Design review of the part built by this model. Coordinates are the model's own, in mm. A direction names the side the tool comes from. Coordinates: 2 decimals unless noted, no trailing zeros. Loops run counter-clockwise (first coordinate to the right, second up) from the corner with the lowest first, then second, coordinate; pieces in that order, holes last. Notation, with made-up numbers: (14, -33) -> (42, -33) arc R28 cw to (42, 2) -> close; hole circle Ø7 at (30.25, 31.5). An arc over 180 degrees is marked (long way). Answer in a Markdown table with one row per item.
```python
from build123d import *

# Parameters (mm, degrees)
BOSS_EXTRUDE1_DEPTH = 19.05
CUT_EXTRUDE1_START  = -3.175
CUT_EXTRUDE1_DEPTH  = 3.175


# Read off the part's stored shape, not the designer's step: Cut-Extrude1
with BuildPart() as part:
    # Sketch1 → Boss-Extrude1 (new body)
    with BuildSketch(Plane.XY):
        with BuildLine():
            Line((157.234081882, 128.980548454), (152.224173193, 179.795336584))
            Line((152.224173193, 179.795336584), (161.70321507, 180.729890008))
            Line((161.70321507, 180.729890008), (166.6875, 130.175))
            add(Edge.make_bspline(
                [(0, 0), (73.666580622, 1.740675992), (181.188092361, 36.200835609), (166.6875, 130.175)],
                knots=[0, 0, 0, 0, 1, 1, 1, 1], degree=3))
            add(Edge.make_bspline(
                [(0, 0), (-73.666580622, 1.740675992), (-181.188092361, 36.200835609), (-166.6875, 130.175)],
                knots=[0, 0, 0, 0, 1, 1, 1, 1], degree=3))
            Line((-166.6875, 130.175), (-111.860365766, 686.278790089))
            Line((-111.860365766, 686.278790089), (-102.381323889, 685.344236665))
            Line((-102.381323889, 685.344236665), (-157.234081882, 128.980548454))
            add(Edge.make_bspline(
                [(0, 9.52776174), (-1.117611602, 9.555193192), (-3.340472897, 9.624755056), (-7.880039481, 9.827207732), (-13.652210416, 10.198958437), (-20.725459036, 10.840441372), (-30.303235723, 11.962316267), (-42.47749757, 13.875858033), (-57.165232888, 17.02314898), (-71.689613059, 21.050850851), (-90.515854195, 27.626537064), (-112.436111514, 38.157452487), (-130.643933928, 51.803557723), (-142.189146149, 64.564536934), (-149.192253507, 75.075537554), (-153.541361304, 84.674022673), (-156.058613173, 92.923629982), (-157.442658539, 99.418206789), (-158.29640922, 106.242287005), (-158.540175044, 112.221426054), (-158.437150466, 117.190167219), (-158.20642164, 121.010360535), (-157.881730698, 124.277278241), (-157.584058118, 126.601085874), (-157.415798733, 127.781927866), (-157.316566229, 128.446705395), (-157.261207353, 128.804756083), (-157.234081882, 128.980548454)],
                knots=[0.001057036, 0.001057036, 0.001057036, 0.001057036, 0.016679825, 0.032302613, 0.063548191, 0.094793768, 0.126039346, 0.1885305, 0.251021655, 0.31351281, 0.376003965, 0.500986274, 0.625968584, 0.688459739, 0.750950893, 0.813442048, 0.844687626, 0.875933203, 0.90717878, 0.938424358, 0.954047147, 0.969669935, 0.985292724, 0.993104118, 0.997009815, 0.998962664, 1.000915513, 1.000915513, 1.000915513, 1.000915513], degree=3))
            add(Edge.make_bspline(
                [(157.234081882, 128.980548454), (157.261207353, 128.804756083), (157.316566229, 128.446705395), (157.415798733, 127.781927866), (157.584058118, 126.601085874), (157.881730698, 124.277278241), (158.20642164, 121.010360535), (158.437150466, 117.190167219), (158.540175044, 112.221426054), (158.29640922, 106.242287005), (157.442658539, 99.418206789), (156.058613173, 92.923629982), (153.541361304, 84.674022673), (149.192253507, 75.075537554), (142.189146149, 64.564536934), (130.643933928, 51.803557723), (112.436111514, 38.157452487), (90.515854195, 27.626537064), (71.689613059, 21.050850851), (57.165232888, 17.02314898), (42.47749757, 13.875858033), (30.303235723, 11.962316267), (20.725459036, 10.840441372), (13.652210416, 10.198958437), (7.880039481, 9.827207732), (3.340472897, 9.624755056), (1.117611602, 9.555193192), (0, 9.52776174)],
                knots=[0.001057036, 0.001057036, 0.001057036, 0.001057036, 0.003009885, 0.004962733, 0.00886843, 0.016679825, 0.032302613, 0.047925402, 0.063548191, 0.094793768, 0.126039346, 0.157284923, 0.1885305, 0.251021655, 0.31351281, 0.376003965, 0.500986274, 0.625968584, 0.688459739, 0.750950893, 0.813442048, 0.875933203, 0.90717878, 0.938424358, 0.969669935, 0.985292724, 1.000915513, 1.000915513, 1.000915513, 1.000915513], degree=3))
        make_face()
    extrude(amount=BOSS_EXTRUDE1_DEPTH)

    # Cut-Extrude1 outline → Cut-Extrude1 (cut)
    with BuildSketch(Plane.XY.offset(19.05).offset(CUT_EXTRUDE1_START)):
        with BuildLine():
            Line((-107.13348355, 685.812759448), (-161.973395498, 129.579366829))
            add(Edge.make_bspline(
                [(-161.973395498, 129.579366829), (-162.00171525, 129.395834674), (-162.028495082, 129.221667618), (-162.081541528, 128.869683844), (-162.159761136, 128.342436218), (-162.332851825, 127.117281326), (-162.641575692, 124.687275119), (-162.842770083, 122.639027203), (-163.16267738, 118.588121623), (-163.265984358, 115.948323615), (-163.262423556, 108.206156668), (-162.842404671, 103.28119599), (-161.248767489, 93.87057237), (-160.075199693, 89.384607046), (-157.045094148, 80.81595139), (-155.188366146, 76.733021658), (-150.853165213, 68.941465452), (-148.374445898, 65.232835538), (-142.854480948, 58.172008914), (-139.813114246, 54.819957421), (-129.940113205, 45.284353516), (-122.357367523, 39.621644841), (-105.759630554, 29.639229241), (-96.746229237, 25.320471564), (-77.904058281, 17.968013466), (-68.075890669, 14.934086027), (-48.230630184, 10.070216513), (-38.213566045, 8.240058869), (-18.618837768, 5.689359978), (-9.040867048, 4.96882986), (0, 4.751150948)],
                knots=[0, 0, 0, 0, 0.001953125, 0.001953125, 0.00390625, 0.0078125, 0.015625, 0.03125, 0.03125, 0.0625, 0.0625, 0.125, 0.125, 0.1875, 0.1875, 0.25, 0.25, 0.3125, 0.3125, 0.375, 0.375, 0.5, 0.5, 0.625, 0.625, 0.75, 0.75, 0.875, 0.875, 1, 1, 1, 1], degree=3))
            add(Edge.make_bspline(
                [(0, 4.751150948), (9.040867048, 4.96882986), (18.618837768, 5.689359978), (38.213566045, 8.240058869), (48.230630184, 10.070216513), (68.075890669, 14.934086027), (77.904058281, 17.968013466), (96.746229237, 25.320471564), (105.759630554, 29.639229241), (122.357367523, 39.621644841), (129.940113205, 45.284353516), (139.813114246, 54.819957421), (142.854480948, 58.172008914), (148.374445898, 65.232835538), (150.853165213, 68.941465452), (155.188366146, 76.733021658), (157.045094148, 80.81595139), (160.075199693, 89.384607046), (161.248767489, 93.87057237), (162.842404671, 103.28119599), (163.262423556, 108.206156668), (163.265984358, 115.948323615), (163.16267738, 118.588121623), (162.842770083, 122.639027203), (162.708640489, 124.004525814), (162.465162127, 126.075850353), (162.332851825, 127.117281326), (162.159761136, 128.342436218), (162.081541528, 128.869683844), (162.028495082, 129.221667618), (162.00171525, 129.395834674), (161.973395498, 129.579366829)],
                knots=[0, 0, 0, 0, 0.125, 0.125, 0.25, 0.25, 0.375, 0.375, 0.5, 0.5, 0.625, 0.625, 0.6875, 0.6875, 0.75, 0.75, 0.8125, 0.8125, 0.875, 0.875, 0.9375, 0.9375, 0.96875, 0.96875, 0.984375, 0.984375, 0.9921875, 0.99609375, 0.998046875, 0.998046875, 1, 1, 1, 1], degree=3))
            Line((161.973395498, 129.579366829), (156.976332854, 180.263859367))
            Line((156.976332854, 180.263859367), (152.224173193, 179.795336584))
            Line((152.224173193, 179.795336584), (157.234081882, 128.980548454))
            add(Edge.make_bspline(
                [(157.234081882, 128.980548454), (157.261207353, 128.804756083), (157.316566229, 128.446705395), (157.415798733, 127.781927866), (157.584058118, 126.601085874), (157.881730698, 124.277278241), (158.20642164, 121.010360535), (158.437150466, 117.190167219), (158.540175044, 112.221426054), (158.29640922, 106.242287005), (157.442658539, 99.418206789), (156.058613173, 92.923629982), (153.541361304, 84.674022673), (149.192253507, 75.075537554), (142.189146149, 64.564536934), (130.643933928, 51.803557723), (112.436111514, 38.157452487), (90.515854195, 27.626537064), (71.689613059, 21.050850851), (57.165232888, 17.02314898), (42.47749757, 13.875858033), (30.303235723, 11.962316267), (20.725459036, 10.840441372), (13.652210416, 10.198958437), (7.880039481, 9.827207732), (3.340472897, 9.624755056), (1.117611602, 9.555193192), (0, 9.52776174)],
                knots=[0.001057036, 0.001057036, 0.001057036, 0.001057036, 0.003009885, 0.004962733, 0.00886843, 0.016679825, 0.032302613, 0.047925402, 0.063548191, 0.094793768, 0.126039346, 0.157284923, 0.1885305, 0.251021655, 0.31351281, 0.376003965, 0.500986274, 0.625968584, 0.688459739, 0.750950893, 0.813442048, 0.875933203, 0.90717878, 0.938424358, 0.969669935, 0.985292724, 1.000915513, 1.000915513, 1.000915513, 1.000915513], degree=3))
            add(Edge.make_bspline(
                [(0, 9.52776174), (-1.117611602, 9.555193192), (-3.340472897, 9.624755056), (-7.880039481, 9.827207732), (-13.652210416, 10.198958437), (-20.725459036, 10.840441372), (-30.303235723, 11.962316267), (-42.47749757, 13.875858033), (-57.165232888, 17.02314898), (-71.689613059, 21.050850851), (-90.515854195, 27.626537064), (-112.436111514, 38.157452487), (-130.643933928, 51.803557723), (-142.189146149, 64.564536934), (-149.192253507, 75.075537554), (-153.541361304, 84.674022673), (-156.058613173, 92.923629982), (-157.442658539, 99.418206789), (-158.29640922, 106.242287005), (-158.540175044, 112.221426054), (-158.437150466, 117.190167219), (-158.20642164, 121.010360535), (-157.881730698, 124.277278241), (-157.584058118, 126.601085874), (-157.415798733, 127.781927866), (-157.316566229, 128.446705395), (-157.261207353, 128.804756083), (-157.234081882, 128.980548454)],
                knots=[0.001057036, 0.001057036, 0.001057036, 0.001057036, 0.016679825, 0.032302613, 0.063548191, 0.094793768, 0.126039346, 0.1885305, 0.251021655, 0.31351281, 0.376003965, 0.500986274, 0.625968584, 0.688459739, 0.750950893, 0.813442048, 0.844687626, 0.875933203, 0.90717878, 0.938424358, 0.954047147, 0.969669935, 0.985292724, 0.993104118, 0.997009815, 0.998962664, 1.000915513, 1.000915513, 1.000915513, 1.000915513], degree=3))
            Line((-157.234081882, 128.980548454), (-102.381323889, 685.344236665))
            Line((-102.381323889, 685.344236665), (-107.13348355, 685.812759448))
        make_face()
    extrude(amount=CUT_EXTRUDE1_DEPTH, mode=Mode.SUBTRACT)


solid = part.part
```
(1) Draft analysis for pull direction Y (two halves, no side actions). For faces 1 (the flat face through (-139.66, 404.33, 9.39)), 2 (the flat face through (-134.17, 411.59, 17.44)), 3 (the flat face through (-147, 294, 19.05)), state which applies: pulls with the +Y half, pulls with the -Y half, needs draft (parallel to the pull), parting line crosses it, or undercut.
Evaluation:
| item | result |
|---|---|
| face 1 | pulls with the +Y half |
| face 2 | undercut |
| face 3 | needs draft |
(2) Take a section at A-A on y = 414.5. Give the boundary of the cut face in (x, z) (3 decimals).
Evaluation:
| item | result |
|---|---|
| outline | (-138.655, 0) -> (-129.084, 0) -> (-129.084, 15.875) -> (-133.883, 15.875) -> (-133.883, 19.05) -> (-138.655, 19.05) -> close |
(3) Tool access review of faces 4 (the flat face through (154.764, 154.032, 7.826)), 5 (the flat face through (164.16, 155.81, 9.39)), 6 (the flat face through (-146, 246, 15.875)): name each direction out of +Z, -Z, +X, -X, +Y, -Y from which nothing blocks a thin tool from reaching the whole face with its end or side.
Evaluation:
| item | result |
|---|---|
| face 4 | +Z, -Z |
| face 5 | +Z, -Z, +X, +Y |
| face 6 | +Z |
(4) For pin 1 (8 mm diameter, centred on y = 219.5, z = 9, fed in from -X); pin 2 (6 mm diameter, centred on x = 118.5, z = 2, fed in from -Y), all flat-tipped, find the tip position at first contact; note any pin that passes through.
Evaluation:
| item | result |
|---|---|
| pin 1 | stops at x = -158.28 |
| pin 2 | stops at y = 29.96 |
(5) To check wall thickness, follow probe 1 along X at (y, z) = (70.5, 6.75); probe 2 along X at (y, z) = (40, 5.25); probe 3 along X at (y, z) = (478, 9.5). State the ranges of each line that lie inside material, in increasing order.
Evaluation:
| item | result |
|---|---|
| probe 1 | x = -157.16 to -146.04, 146.04 to 157.16 |
| probe 2 | x = -130.32 to -113.68, 113.68 to 130.32 |
| probe 3 | x = -132.39 to -122.82 |
